The model under review builds one solid part; all positions refer to its coordinate system, in mm. Face numbers are marked on the shaded views. A direction names the side the tool comes from. Give positions to 0.01 mm unless a question says otherwise; leave off trailing zeros. Write each loop counter-clockwise with the first axis right and the second up, starting at its lowest first coordinate (ties: lowest second). Pieces come first, ordered by that corner, then holes. Notation, with made-up numbers: (-24.5, 43) -> (-1.5, 43) arc R13 ccw to (-1.5, 62) -> close; hole circle Ø7 at (60, 25). An arc over 180 degrees is marked (long way). Use CSV: the item, a comma, the result in double quotes.
```python
from build123d import *

# Parameters (mm, degrees)
F0_R     = 22.982221
F0_R_2   = 12.037169
F1_DEPTH = 25
F2_R     = 4.502858
F3_DEPTH = 22.983221
F4_R     = 4.066018
F5_DEPTH = 22.983221


with BuildPart() as f1:
    # F0 (on Top) → F1 (new body)
    with BuildSketch(Plane.XY):
        Circle(F0_R)
        Circle(F0_R_2, mode=Mode.SUBTRACT)
    extrude(amount=F1_DEPTH)

    # F2 (on Right) → F3 (cut, through all)
    with BuildSketch(Plane.YZ):
        with Locations((0, 17.034575)):
            Circle(F2_R)
    extrude(amount=-F3_DEPTH, mode=Mode.SUBTRACT)

    # F4 (on Front) → F5 (cut, through all)
    with BuildSketch(Plane.XZ):
        with Locations((0, 13.683511)):
            Circle(F4_R)
    extrude(amount=F5_DEPTH, mode=Mode.SUBTRACT)


solid = f1.part
```
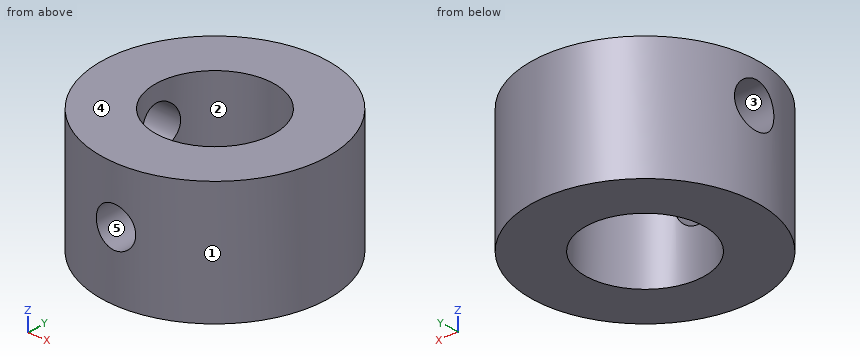
Q1. Insertion check: pin 1 (1.5 mm diameter, centred on y = -17.5, z = 17, fed in from -X); pin 2 (2 mm diameter, centred on y = -2.5, z = 5, fed in from -X); pin 3 (3 mm diameter, centred on x = 14, z = 11.5, fed in from -Y); pin 4 (21.5 mm diameter, centred on x = 0, y = 0, fed in from +Z) (3 decimals). Each pin has a flat end and moves straight along its axis. Give the tip position at first contact, or say it passes through.
Derived:
pin 1,"stops at x = -15.74"
pin 2,"stops at x = -22.93"
pin 3,"stops at y = -19.29"
pin 4,"passes through"
Q2. Consider section A-A (y = 0). Write out the cut boundary in (x, z).
Derived:
outline,"(-22.98, 0) -> (-12.04, 0) -> (-12.04, 12.53) -> (-22.98, 12.53) -> close; (-22.98, 21.54) -> (-12.04, 21.54) -> (-12.04, 25) -> (-22.98, 25) -> close; (12.04, 0) -> (22.98, 0) -> (22.98, 25) -> (12.04, 25) -> close"
Q3. Consider section D-D (x = -8). Write out the cut boundary in (y, z).
Derived:
outline,"(-21.54, 0) -> (-8.99, 0) -> (-8.99, 25) -> (-21.54, 25) -> close; (8.99, 0) -> (21.54, 0) -> (21.54, 25) -> (8.99, 25) -> close"
Q4. Consider section C-C (z = 7.75). Write out the cut boundary in (x, y).
Derived:
outline,"circle Ø45.96 at (0, 0); hole circle Ø24.07 at (0, 0)"
Q5. The part is to be moulded in two halves that separate along X. For the marked faces 1, 2 and 3, say which applies: pulls with the +X half, pulls with the -X half, needs draft (parallel to the pull), parting line crosses it, or undercut.
Derived:
face 1,"parting line crosses it"
face 2,"undercut"
face 3,"needs draft"
Q6. To check wall thickness, follow probe 1 along X at (y, z) = (0, 9.75); probe 2 along Z at (x, y) = (0, -16). State the ranges of each line that lie inside material, in increasing order.
Derived:
probe 1,"x = -22.98 to -12.04, 12.04 to 22.98"
probe 2,"z = 0 to 9.62, 17.75 to 25"
Q7. Machinability: for the marked faces 4 and 5, which of the approach directions +Z, -Z, +X, -X, +Y, -Y give a long, thin tool a straight path to every point of the face, cutting with its end or side? Answer none if there is none.
Derived:
face 4,"+Z, +X, -X, +Y, -Y"
face 5,"-Y"
Q8. Consider section B-B (x = 0). Write out the cut boundary in (y, z), then the cut area to 3 significant figures.
Derived:
outline,"(-22.98, 0) -> (-12.04, 0) -> (-12.04, 9.62) -> (-22.98, 9.62) -> close; (-22.98, 17.75) -> (-12.04, 17.75) -> (-12.04, 25) -> (-22.98, 25) -> close; (12.04, 0) -> (22.98, 0) -> (22.98, 25) -> (12.04, 25) -> close"
area,"458 mm2"
